The listing builds one solid part. Answer for the finished solid, in the listing's coordinates (mm). Face numbers are marked on the shaded views. A direction names the side the tool comes from. Round coordinates to 2 decimals unless told otherwise and drop trailing zeros. Write each loop counter-clockwise with the first axis right and the second up, starting at its lowest first coordinate (ties: lowest second). Pieces come first, ordered by that corner, then holes. Notation, with made-up numbers: M 10,24 L 20,24 A14 cw 20,48 Z; hole C 21.25,17.25 d2. An arc over 180 degrees is marked long. One line per item, written item: value. Start each with the question number.
(1) Consider probe 1 along X at (y, z) = (-3.5, 3); probe 2 along Y at (x, z) = (1.75, 18.5); probe 3 along Z at (x, y) = (2.5, 103). Determine where each line is inside the solid, lowest interval first.
(2) Given P1, Ø6, axis at x = 7.5, y = -8.5, coming from the +Z side; P2, Ø2, axis at x = -2, z = 12.5, coming from the -Y side; P3, Ø1.2, axis at x = 2, y = -26.5, coming from the +Z side, each flat-ended and moving along its own axis, determine where each tip first touches the part or whether it passes through.
(3) Section C-C (z = 17.25) is taken. Determine the outline of the cut face in (x, y).
(4) Section B-B (z = 6) is taken. Determine the outline of the cut face in (x, y).
(5) For the marked faces 4 and 5, determine the directions among +Z, -Z, +X, -X, +Y, -Y from which every point of the face is accessible in a straight line to the end or side of a thin tool.
(6) Section A-A (y = 45) is taken. Determine the outline of the cut face in (x, z).
(7) For a pull along X with two mould halves and no side action, classify the marked faces 1, 2 and 3 as released by +X, released by -X, zero draft, split by the parting line, or undercut.
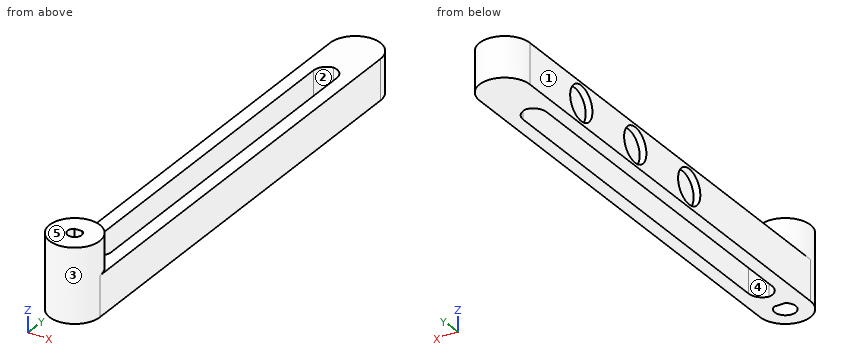
```python
from build123d import *

# Parameters (mm, degrees)
BOSS_EXTRUDE1_DEPTH = 12
SKETCH2_R           = 3.1
BOSS_EXTRUDE2_DEPTH = 15
CUT_EXTRUDE1_START  = -50
CUT_EXTRUDE1_DEPTH  = 50
CUT_EXTRUDE2_START  = -15
CUT_EXTRUDE2_DEPTH  = 15
SKETCH5_W           = 7
SKETCH5_H           = 112.5
CUT_EXTRUDE3_DEPTH  = 12
SKETCH6_R           = 5.15
CUT_EXTRUDE4_DEPTH  = 2
FILLET1_R           = 4
BOSS_EXTRUDE3_DEPTH = 10
SKETCH9_R           = 2.1
CUT_EXTRUDE5_DEPTH  = 7
BOSS_EXTRUDE4_DEPTH = 7


with BuildPart() as part:
    # Sketch1 → Boss-Extrude1 (new body)
    with BuildSketch(Plane.XY):
        with BuildLine():
            Line((-5.64516129, 102.580645161), (-5.64516129, -27.419354839))
            ThreePointArc((-5.64516129, -27.419354839), (1.85483871, -34.919354839), (9.35483871, -27.419354839))
            Line((9.35483871, -27.419354839), (9.35483871, 102.580645161))
            ThreePointArc((9.35483871, 102.580645161), (1.85483871, 110.080645161), (-5.64516129, 102.580645161))
        make_face()
    extrude(amount=BOSS_EXTRUDE1_DEPTH)

    # Sketch2 → Boss-Extrude2 (add)
    with BuildSketch(Plane.XY.offset(12)):
        with Locations(Location((1.85483871, -27.419354839, 0), (0, 0, 180))):
            Circle(SKETCH2_R)
    extrude(amount=BOSS_EXTRUDE2_DEPTH)

    # Sketch3 → Cut-Extrude1 (cut)
    with BuildSketch(Plane.XY.offset(27).offset(CUT_EXTRUDE1_START)):
        with BuildLine():
            Line((0.166644408, -24.819354839), (3.543033011, -24.819354839))
            ThreePointArc((3.543033011, -24.819354839), (1.85483871, -30.519354839), (0.166644408, -24.819354839))
        make_face()
    extrude(amount=CUT_EXTRUDE1_DEPTH, mode=Mode.SUBTRACT)

    # Sketch4 → Cut-Extrude2 (cut)
    with BuildSketch(Plane.XY.offset(27).offset(CUT_EXTRUDE2_START)):
        with BuildLine():
            Line((0.166644408, -24.819354839), (3.543033011, -24.819354839))
            ThreePointArc((3.543033011, -24.819354839), (1.85483871, -24.319354839), (0.166644408, -24.819354839))
        make_face()
    extrude(amount=CUT_EXTRUDE2_DEPTH, mode=Mode.SUBTRACT)

    # Sketch5 → Cut-Extrude3 (cut)
    with BuildSketch(Plane.XY.offset(12)):
        with Locations((1.85483871, 36.330645161)):
            Rectangle(SKETCH5_W, SKETCH5_H)
    extrude(amount=-CUT_EXTRUDE3_DEPTH, mode=Mode.SUBTRACT)

    # Sketch6 → Cut-Extrude4 (cut)
    with BuildSketch(Plane.ZY.offset(5.64516129)):
        with Locations(Location((6, 78.768969581, 0), (0, 0, 270))):
            Circle(SKETCH6_R)
        with Locations(Location((6, 53.768969581, 0), (0, 0, 270))):
            Circle(SKETCH6_R)
        with Locations(Location((6, 28.768969581, 0), (0, 0, 270))):
            Circle(SKETCH6_R)
    extrude(amount=-CUT_EXTRUDE4_DEPTH, mode=Mode.SUBTRACT)

    # Fillet1
    # the kernel refuses this fillet: 4 mm, written as the material it adds along each edge
    with BuildSketch(Plane(origin=(-1.64516129, -19.919354839, 12), x_dir=(0, 1, 0), z_dir=(0, 0, -1)), Plane(origin=(5.35483871, -19.919354839, 12), x_dir=(-1, 0, 0), z_dir=(0, 0, -1)), Plane(origin=(5.35483871, 92.580645161, 12), x_dir=(0, -1, 0), z_dir=(0, 0, -1))) as fillet1_piece_1:
        with BuildLine():
            CenterArc((FILLET1_R, FILLET1_R), FILLET1_R, 180, 90)
            Line((0, FILLET1_R), (0, 0))
            Line((0, 0), (FILLET1_R, 0))
        make_face()
    extrude(amount=12)
    with BuildSketch(Plane(origin=(-1.64516129, 92.580645161, 12), x_dir=(0, -1, 0), z_dir=(0, 0, -1))) as fillet1_piece_2:
        with BuildLine():
            CenterArc((FILLET1_R, -FILLET1_R), FILLET1_R, 90, 90)
            Line((0, -FILLET1_R), (0, 0))
            Line((0, 0), (FILLET1_R, 0))
        make_face()
    extrude(amount=12)

    # Sketch7 → Boss-Extrude3 (add)
    with BuildSketch(Plane.XY.offset(12)):
        with BuildLine():
            ThreePointArc((-5.64516129, -27.419354839), (1.85483871, -34.919354839), (9.35483871, -27.419354839))
            ThreePointArc((9.35483871, -27.419354839), (1.85483871, -19.919354839), (-5.64516129, -27.419354839))
        make_face()
    extrude(amount=BOSS_EXTRUDE3_DEPTH)

    # Sketch9 → Cut-Extrude5 (cut)
    with BuildSketch(Plane.XY.offset(22)):
        with Locations((1.85483871, -27.419354839)):
            Circle(SKETCH9_R)
    extrude(amount=-CUT_EXTRUDE5_DEPTH, mode=Mode.SUBTRACT)

    # Sketch10 → Boss-Extrude4 (add)
    with BuildSketch(Plane.XY.offset(22)):
        with BuildLine():
            Line((0.694020033, -25.669354839), (3.015657386, -25.669354839))
            ThreePointArc((3.015657386, -25.669354839), (1.85483871, -25.319354839), (0.694020033, -25.669354839))
        make_face()
    extrude(amount=-BOSS_EXTRUDE4_DEPTH)


solid = part.part
```
Recorded:
1. probe 1: x = -5.65 to -1.65, 5.35 to 9.35
1. probe 2: y = -34.92 to -29.52, -25.67 to -19.92
1. probe 3: z = 0 to 12
2. P1: stops at z = 12
2. P2: stops at y = -34.35
2. P3: stops at z = 15
3. outline: C 1.85,-27.42 d15; hole M 0.69,-25.67 A2.1 ccw long 3.02,-25.67 Z
4. outline: M -5.65,-27.42 A7.5 ccw 9.35,-27.42 L 9.35,102.58 A7.5 ccw -5.65,102.58 L -5.65,83.92 L -3.65,83.92 L -3.65,73.62 L -5.65,73.62 L -5.65,58.92 L -3.65,58.92 L -3.65,48.62 L -5.65,48.62 L -5.65,33.92 L -3.65,33.92 L -3.65,23.62 L -5.65,23.62 Z; hole M -1.65,-15.92 A4 ccw 1.85,-19.89 A4 ccw 5.35,-15.92 L 5.35,88.58 A4 ccw 1.85,92.55 A4 ccw -1.65,88.58 Z; hole M 0.17,-24.82 A3.1 ccw long 3.54,-24.82 Z
5. face 4: +Z, -Z
5. face 5: +Z, +X, -X, +Y, -Y
6. outline: M -5.65,0 L -1.65,0 L -1.65,12 L -5.65,12 Z; M 5.35,0 L 9.35,0 L 9.35,12 L 5.35,12 Z
7. face 1: released by -X
7. face 2: undercut
7. face 3: split by the parting line
